from build123d import *

# Parameters (mm, degrees)
BASEHEAD_DEPTH      = 5.5
SKETCH4_W           = 0.6
SKETCH4_H           = 11.005553499
BOSS_EXTRUDE1_DEPTH = 6


# Read off the part's stored shape, not the designer's step: HeadChamfer
with BuildPart() as part:
    # Sketch1 → BaseHead (new body)
    with BuildSketch(Plane(origin=(0, 0, 0), x_dir=(0, 0, -1), z_dir=(1, 0, 0))):
        Polygon((6.5, 3.75277675), (6.5, -3.75277675), (0, -7.505553499), (-6.5, -3.75277675), (-6.5, 3.75277675), (0, 7.505553499), align=None)
    extrude(amount=BASEHEAD_DEPTH)

    # HeadChamfer outline → HeadChamfer (revolve, cut)
    with BuildSketch(Plane.YX):
        Polygon((7.505553503, 0.580556586), (6.499999425, -3.32e-07), (7.505553503, -1.347e-06), align=None)
    revolve(axis=Axis((0, 0, 0), (1, 0, 0)), mode=Mode.SUBTRACT)

    # HeadChamfer 2 outline → HeadChamfer 2 (revolve)
    with BuildSketch(Plane.YX):
        Polygon((4, 5.5), (4, 39.8095), (3.3095, 40.5), (0, 40.5), (0, 5.5), align=None)
    revolve(axis=Axis((0, 0, 0), (1, 0, 0)))

    # Sketch4 → BearingFace (revolve, cut)
    with BuildSketch(Plane.XY, mode=Mode.PRIVATE) as bearingface_sk:
        with Locations((5.2, 12.00277675)):
            Rectangle(SKETCH4_W, SKETCH4_H)
    revolve(bearingface_sk.sketch.rotate(Axis((0, 0, 0), (1, 0, 0)), 90), axis=Axis((0, 0, 0), (1, 0, 0)), mode=Mode.SUBTRACT)

    # Sketch5 → Boss-Extrude1 (add)
    with BuildSketch(Plane(origin=(35.5, 0, 0), x_dir=(0, 0, -1), z_dir=(1, 0, 0))):
        Polygon((-3.043097903, 6.86096848), (-7.46332195, 0.79508415), (-4.420224047, -6.06588433), (3.043097903, -6.86096848), (7.46332195, -0.79508415), (4.420224047, 6.06588433), align=None)
    extrude(amount=-BOSS_EXTRUDE1_DEPTH)


solid = part.part
Build history of the part. All positions in model axes, mm. A direction names the side the tool comes from. Coordinates: 2 decimals unless noted, no trailing zeros. Order: outer loops, then holes, each group sorted by start corner. A loop starts at its lowest first (then second) coordinate and runs counter-clockwise, first axis right, second up. Notation, with made-up numbers: M -22.5,89 L 6.5,89 A21 cw 6.5,102 Z; hole C 71,-19 d3. An arc over 180 degrees is marked long. One line per question, with ' | ' between items. Start each with the question number.
Q1. Probe L1, parallel to X at y = -5.25, z = 2.5; L2, parallel to Z at x = 23.5, y = 2.25; L3, parallel to X at y = -5.5, z = -3.75. List the from-to ranges inside material, lowest first. Write a range as from..to.
Q2. Flat gauge pins, fed straight in: pin 1 Ø1.5 at (y, z) = (2.5, 4) entering from +X; pin 2 Ø5 at (x, z) = (34, -5.5) entering from +Y; pin 3 Ø1 at (x, z) = (10.5, -0.5) entering from -Y; pin 4 Ø4 at (y, z) = (5.5, -4) entering from -X. Where does each tip first touch, or does it go through?
Q3. 3-axis set-ups, long thin cutter, end or side, ignore diameter. For faces 1 (the face through (2.4, -5.6, -3.3)), 2 (the face through (2, 0, 6.5)), 3 (the face through (4.9, -3, -6)), 4 (the face through (32.542, 6.458, -0.741)), 5 (the face through (2.4, 5.6, 3.3)): which of +Z, -Z, +X, -X, +Y, -Y reach the whole face in a straight line?
Q4. Saw through at A-A (x = 4.5). List the corners of the cut face in (y, z), then the cut area to 3 significant figures.
Q5. Two-plate mould, pull along X, no slides. Class faces 6 (the face through (4.9, 7, 0)), 7 (the face through (35.5, -3, 3)), 8 (the face through (0, 0, 0)), 9 (the face through (32.54, -2.59, 5.96)): +X half, -X half, draft (parallel to the pull), parting line (faces both ways), or undercut.
Q6. Saw through at B-B (x = 9). List the corners of the cut face in (y, z).
Check values:
1) L1: x = 0..5.5, 29.5..35.5 | L2: z = -3.31..3.31 | L3: x = 29.5..35.5
2) pin 1: stops at x = 39.84 | pin 2: stops at y = 6.22 | pin 3: stops at y = -4 | pin 4: stops at x = 0
3) face 1: -Z, -X, -Y | face 2: +Z, -X, +Y, -Y | face 3: -Z, -Y | face 4: -Z, +X, +Y | face 5: +Z, -X, +Y
4) outline: M -7.51,0 L -3.75,-6.5 L 3.75,-6.5 L 7.51,0 L 3.75,6.5 L -3.75,6.5 Z | area: 146 mm2
5) face 6: undercut | face 7: +X half | face 8: -X half | face 9: draft
6) outline: C 0,0 d8
